Verification items for this drawing (mm, ordinates from the low corner). Round coordinates to 2 decimals unless told otherwise and drop trailing zeros. Loops run counter-clockwise (first coordinate to the right, second up) from the corner with the lowest first, then second, coordinate; pieces in that order, holes last. Notation, with made-up numbers: M 79.5,77.25 L 117.5,77.25 A9 ccw 117.5,90.25 Z; hole C 78,26 d7. An arc over 180 degrees is marked long. Write item = value, one per line. Start each with the question number.
(1) Cross-section at D-D on x = 4. Record the boundary of the cut face in (y, z), plus the area to 3 significant figures.
(2) Cross-section at B-B on x = 3.3. Record the boundary of the cut face in (y, z).
(3) Cross-section at A-A on z = 7. Record the boundary of the cut face in (x, y), plus the area to 3 significant figures.
(4) Scan lines: L1, parallel to X at y = 3.45, z = 7.4; L2, parallel to Y at x = 3.3, z = 7.2; L3, parallel to Z at x = 4.75, y = 3.25. Record each from-to range of solid material in increasing order. Write a range as from..to.
(5) Go/stop test with a flat-tipped pin: P1, Ø0.5, axis at x = 4, y = 4, coming from the +Z side. Record where the tip stops, or that it passes through.
(6) Cross-section at C-C on y = 2.84. Record the boundary of the cut face in (x, z).
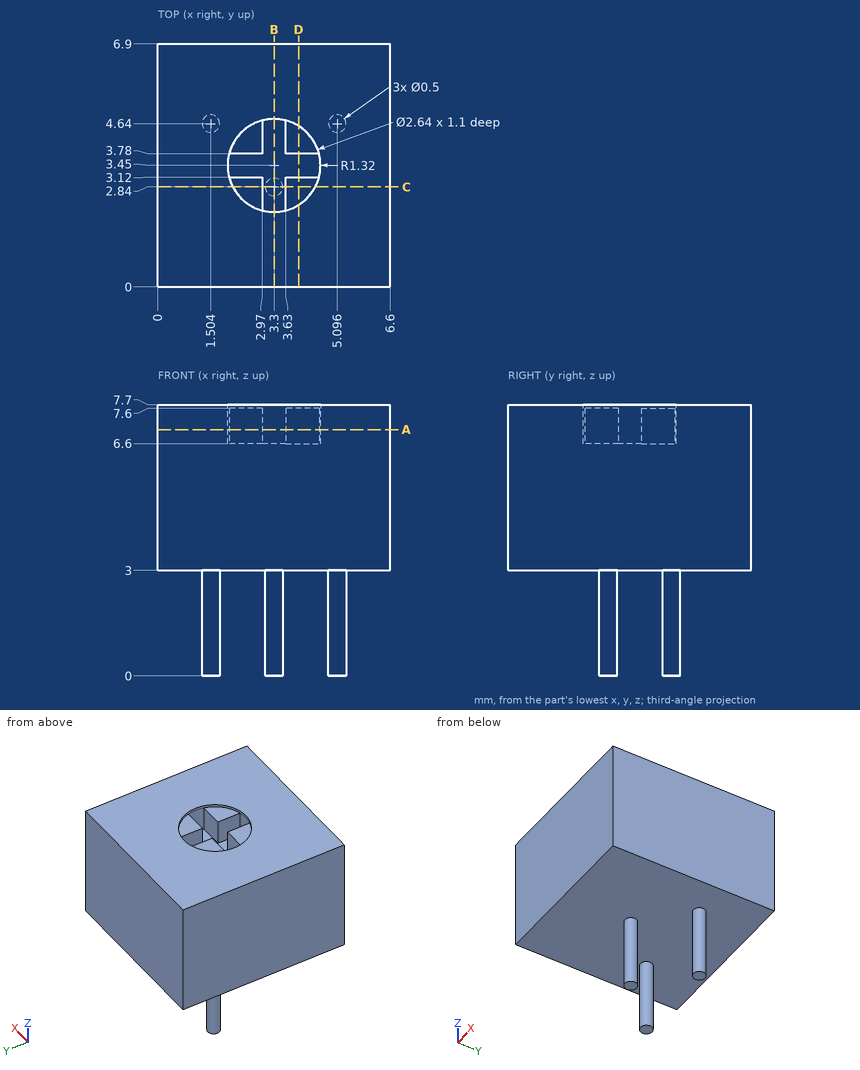
Result:
q1.outline = M 0,3 L 6.9,3 L 6.9,7.7 L 4.57,7.7 L 4.57,7.6 L 3.78,7.6 L 3.78,6.6 L 3.12,6.6 L 3.12,7.6 L 2.33,7.6 L 2.33,7.7 L 0,7.7 Z
q1.area = 31.5 mm^2
q2.outline = M 0,3 L 2.59,3 L 2.59,0 L 3.09,0 L 3.09,3 L 6.9,3 L 6.9,7.7 L 4.77,7.7 L 4.77,6.6 L 2.13,6.6 L 2.13,7.7 L 0,7.7 Z
q3.outline = M 0,0 L 6.6,0 L 6.6,6.9 L 0,6.9 Z; hole M 2.02,3.12 L 2.97,3.12 L 2.97,2.17 A1.32 ccw 3.63,2.17 L 3.63,3.12 L 4.58,3.12 A1.32 ccw 4.58,3.78 L 3.63,3.78 L 3.63,4.73 A1.32 ccw 2.97,4.73 L 2.97,3.78 L 2.02,3.78 A1.32 ccw Z
q3.area = 42.5 mm^2
q4.L1 = 0..1.98, 4.62..6.6
q4.L2 = 0..2.13, 4.77..6.9
q4.L3 = 3..7.7
q5.P1 = 7.6
q6.outline = M 0,3 L 3.05,3 L 3.05,0 L 3.55,0 L 3.55,3 L 6.6,3 L 6.6,7.7 L 4.47,7.7 L 4.47,7.6 L 3.63,7.6 L 3.63,6.6 L 2.97,6.6 L 2.97,7.6 L 2.13,7.6 L 2.13,7.7 L 0,7.7 Z
